from build123d import *

# Parameters (mm, degrees)
SKETCH1_R           = 2.8
BOSS_EXTRUDE1_DEPTH = 1.5
SKETCH2_R           = 2.25
BOSS_EXTRUDE2_DEPTH = 7
SKETCH3_R           = 2.25
BOSS_EXTRUDE3_DEPTH = 7
CUT_EXTRUDE1_DEPTH  = 103.8
SKETCH5_R           = 1.75
CUT_EXTRUDE2_DEPTH  = 108.0000001


with BuildPart() as part:
    # Sketch1 → Boss-Extrude1 (new body)
    with BuildSketch(Plane(origin=(0, 0, 0), x_dir=(1, 0, 0), z_dir=(0, 1, 0))):
        Circle(SKETCH1_R)
    extrude(amount=BOSS_EXTRUDE1_DEPTH)

    # Sketch2 → Boss-Extrude2 (add)
    with BuildSketch(Plane(origin=(0, 1.5, 0), x_dir=(1, 0, 0), z_dir=(0, 1, 0))):
        Circle(SKETCH2_R)
    extrude(amount=BOSS_EXTRUDE2_DEPTH)

    # Sketch3 → Boss-Extrude3 (add)
    with BuildSketch(Plane.XZ):
        Circle(SKETCH3_R)
    extrude(amount=BOSS_EXTRUDE3_DEPTH)

    # Sketch4 → Cut-Extrude1 (cut, through all)
    with BuildSketch(Plane(origin=(100, 0, 0), x_dir=(0, 0, -1), z_dir=(1, 0, 0))):
        with BuildLine():
            Line((-0.5, 5.5), (-0.5, 8.5))
            ThreePointArc((-0.5, 8.5), (0, 9), (0.5, 8.5))
            Line((0.5, 8.5), (0.5, 5.5))
            ThreePointArc((0.5, 5.5), (0, 5), (-0.5, 5.5))
        make_face()
        with BuildLine():
            Line((0.5, -4), (0.5, -7))
            ThreePointArc((0.5, -7), (0, -7.5), (-0.5, -7))
            Line((-0.5, -7), (-0.5, -4))
            ThreePointArc((-0.5, -4), (0, -3.5), (0.5, -4))
        make_face()
    extrude(amount=-CUT_EXTRUDE1_DEPTH, mode=Mode.SUBTRACT)

    # Sketch5 → Cut-Extrude2 (cut, through all)
    with BuildSketch(Plane(origin=(0, 100, 0), x_dir=(1, 0, 0), z_dir=(0, 1, 0))):
        Circle(SKETCH5_R)
    extrude(amount=-CUT_EXTRUDE2_DEPTH, mode=Mode.SUBTRACT)


solid = part.part
Work out the finished part from the listing and answer in its coordinate system (mm). A direction names the side the tool comes from. Give positions to 0.01 mm unless a question says otherwise; leave off trailing zeros. Order: outer loops, then holes, each group sorted by start corner. A loop starts at its lowest first (then second) coordinate and runs counter-clockwise, first axis right, second up. Notation, with made-up numbers: M 23,-33.75 L 31,-33.75 A21 ccw 31,-7.75 Z; hole C -3.75,-31 d3. An arc over 180 degrees is marked long. Return JSON: item names as keys, results as strings.
Q1. Each of these flat-tipped pins is pushed along its axis until it touches: pin 1 (1 mm diameter, centred on x = 1, y = 0, fed in from -Z) (3 decimals); pin 2 (0.6 mm diameter, centred on x = 2, y = 6.5, fed in from +Z); pin 3 (1.5 mm diameter, centred on x = -1.5, y = 5.5, fed in from +Z). Where does it stop, or does it pass through?
Answer below:
{"pin 1": "stops at z = -2.755", "pin 2": "stops at z = 1.47", "pin 3": "stops at z = 2.12"}
Q2. Find section D-D, the plane x = 2.4. Write down the section's boundary in (y, z), and give its area (3 significant figures).
Answer below:
{"outline": "M 0,-1.44 L 1.5,-1.44 L 1.5,1.44 L 0,1.44 Z", "area": "4.33 mm^2"}
Q3. Find section C-C, the plane y = 1. Write down the section's boundary in (x, z), and give its area (3 significant figures).
Answer below:
{"outline": "C 0,0 d5.6; hole C 0,0 d3.5", "area": "15.0 mm^2"}
Q4. Find section B-B, the plane z = 0. Write down the section's boundary in (x, y).
Answer below:
{"outline": "M -2.8,0 L -2.25,0 L -2.25,-3.5 L -1.75,-3.5 L -1.75,5 L -2.25,5 L -2.25,1.5 L -2.8,1.5 Z; M 1.75,-3.5 L 2.25,-3.5 L 2.25,0 L 2.8,0 L 2.8,1.5 L 2.25,1.5 L 2.25,5 L 1.75,5 Z"}
Q5. Find section A-A, the plane x = 0. Write down the section's boundary in (y, z), and give its area (4 significant figures).
Answer below:
{"outline": "M -7,-2.25 L 0,-2.25 L 0,-2.8 L 1.5,-2.8 L 1.5,-2.25 L 8.5,-2.25 L 8.5,-1.75 L -7,-1.75 Z; M -7,1.75 L 8.5,1.75 L 8.5,2.25 L 1.5,2.25 L 1.5,2.8 L 0,2.8 L 0,2.25 L -7,2.25 Z", "area": "17.15 mm^2"}
Q6. The mould has two halves that part along X. Classify faces 1 (the face through (0, -7, -2)), 2 (the face through (2.146, 4.951, -0.676)), 3 (the face through (1.617, 0.859, 0.67)): pulls with the +X half, pulls with the -X half, needs draft (parallel to the pull), parting line crosses it, or undercut.
Answer below:
{"face 1": "needs draft", "face 2": "parting line crosses it", "face 3": "undercut"}
Q7. Find the intervals of material crossed by line 1 along X through (y, z) = (-1.25, 0); line 2 along Z through (x, y) = (-1.9, -6); line 3 along Y through (x, z) = (1.65, -2.05), in increasing order. Write a range as [from, to].
Answer below:
{"line 1": "x = [-2.25, -1.75], [1.75, 2.25]", "line 2": "z = [-1.21, -0.5], [0.5, 1.21]", "line 3": "y = [0, 1.5]"}
Q8. Which of the six approach directions +Z, -Z, +X, -X, +Y, -Y give full straight-line access (tool end or side, diameter ignored) to faces 4 (the face through (2.146, -3.451, 0.676)), 5 (the face through (-2.8, 0.7, -0.1))?
Answer below:
{"face 4": "-Y", "face 5": "+Y, -Y"}
